Read the model definition and answer for the solid it produces. Units are mm, in the model's axes. A direction names the side the tool comes from. Coordinates: 2 decimals unless noted, no trailing zeros. Loops run counter-clockwise (first coordinate to the right, second up) from the corner with the lowest first, then second, coordinate; pieces in that order, holes last.
from build123d import *

# Parameters (mm, degrees)
SHELL1_T           = -0.8128
FILLET1_R          = 0.508
SKETCH3_W          = 0.762
SKETCH3_H          = 0.762
CUT_EXTRUDE1_DEPTH = 1.016


with BuildPart() as part:
    # Sketch1 → Revolve1 (revolve)
    with BuildSketch(Plane.XY, mode=Mode.PRIVATE) as revolve1_sk:
        with BuildLine():
            Line((0, 0), (0, 14.605))
            ThreePointArc((0, 14.605), (5.588, 14.065513703), (11.176, 14.605))
            Line((11.176, 14.605), (11.176, 0))
            Line((11.176, 0), (0, 0))
        make_face()
    revolve(revolve1_sk.sketch.rotate(Axis((-10.447687892, 0, 0), (1, 0, 0)), 90), axis=Axis((-10.447687892, 0, 0), (1, 0, 0)))

    # Shell1
    shell1_openings = [part.faces().sort_by_distance(p)[0] for p in [
        (0, 0, 0),
        (11.176, 0, 0),
    ]]
    offset(amount=SHELL1_T, openings=shell1_openings, kind=Kind.INTERSECTION)

    # Sketch2 → Revolve2 (revolve)
    with BuildSketch(Plane.XY, mode=Mode.PRIVATE) as revolve2_sk:
        with BuildLine():
            Line((8.636, 13.407835256), (8.636, 11.878888362))
            Line((8.636, 11.878888362), (10.922, 11.878888362))
            Line((10.922, 11.878888362), (10.922, 8.830888362))
            Line((10.922, 8.830888362), (14.732, 8.830888362))
            Line((14.732, 8.830888362), (14.732, 8.38570101))
            Line((14.732, 8.38570101), (10.805439867, 8.38570101))
            Line((10.805439867, 8.38570101), (10.805439867, 7.279783375))
            ThreePointArc((10.805439867, 7.279783375), (10.656650112, 6.92057313), (10.297439867, 6.771783375))
            Line((10.297439867, 6.771783375), (7.757439867, 6.771783375))
            Line((7.757439867, 6.771783375), (7.757439867, 7.279783375))
            Line((7.757439867, 7.279783375), (10.077783765, 7.279783375))
            ThreePointArc((10.077783765, 7.279783375), (10.233104084, 7.344119158), (10.297439867, 7.499439477))
            Line((10.297439867, 7.499439477), (10.297439867, 8.38570101))
            Line((10.297439867, 8.38570101), (6.741439867, 8.38570101))
            Line((6.741439867, 8.38570101), (6.741439867, 8.830888362))
            Line((6.741439867, 8.830888362), (10.297439867, 8.830888362))
            Line((10.297439867, 8.830888362), (10.297439867, 11.412306581))
            Line((10.297439867, 11.412306581), (8.128, 11.412306581))
            Line((8.128, 11.412306581), (8.128, 13.360351664))
            ThreePointArc((8.128, 13.360351664), (8.38210087, 13.383014307), (8.636, 13.407835256))
        make_face()
    revolve(revolve2_sk.sketch.rotate(Axis((-18.402780465, 0, 0), (1, 0, 0)), 90), axis=Axis((-18.402780465, 0, 0), (1, 0, 0)))

    # Fillet1
    fillet1_edges = [part.edges().sort_by_distance(p)[0] for p in [
        (10.922, 0, -11.878888362),
    ]]
    fillet(fillet1_edges, radius=FILLET1_R)

    # Sketch3 → Cut-Extrude1 (cut)
    with BuildSketch(Plane(origin=(10.805439867, 0, 0), x_dir=(0, 0, -1), z_dir=(1, 0, 0))):
        Polygon((4.038854556, 7.665935745), (3.657854556, 7.006024387), (4.317765913, 6.625024387), (4.698765913, 7.284935745), align=None)
        with Locations((0.045782775, 8.277322377)):
            Rectangle(SKETCH3_W, SKETCH3_H)
        Polygon((7.33071852, 4.619467821), (6.670807162, 4.238467821), (7.051807162, 3.578556464), (7.71171852, 3.959556464), align=None)
        with Locations((8.277322377, -0.045782775)):
            Rectangle(SKETCH3_W, SKETCH3_H)
        Polygon((7.665935745, -4.038854556), (7.006024387, -3.657854556), (6.625024387, -4.317765913), (7.284935745, -4.698765913), align=None)
        Polygon((4.619467821, -7.33071852), (4.238467821, -6.670807162), (3.578556464, -7.051807162), (3.959556464, -7.71171852), align=None)
        with Locations((-0.045782775, -8.277322377)):
            Rectangle(SKETCH3_W, SKETCH3_H)
        Polygon((-4.038854556, -7.665935745), (-3.657854556, -7.006024387), (-4.317765913, -6.625024387), (-4.698765913, -7.284935745), align=None)
        Polygon((-7.33071852, -4.619467821), (-6.670807162, -4.238467821), (-7.051807162, -3.578556464), (-7.71171852, -3.959556464), align=None)
        with Locations((-8.277322377, 0.045782775)):
            Rectangle(SKETCH3_W, SKETCH3_H)
        Polygon((-7.665935745, 4.038854556), (-7.006024387, 3.657854556), (-6.625024387, 4.317765913), (-7.284935745, 4.698765913), align=None)
        Polygon((-4.619467821, 7.33071852), (-4.238467821, 6.670807162), (-3.578556464, 7.051807162), (-3.959556464, 7.71171852), align=None)
    extrude(amount=-CUT_EXTRUDE1_DEPTH, mode=Mode.SUBTRACT)


solid = part.part
Q1. Determine the mould class of faces 1 (the face through (9.01, -6.714, -0.882)), 2 (the face through (14.732, 3, 8)) for opening direction Z: +Z half, -Z half, draft (parallel to the pull), parting line (faces both ways), or undercut.
Findings below:
face 1: undercut
face 2: draft
Q2. Flat-ended cylindrical pins translate along their axes: pin 1 Ø4 at (x, y) = (2, -6.5) entering from +Z; pin 2 Ø4 at (x, z) = (10.5, -3) entering from -Y; pin 3 Ø1.5 at (x, z) = (11, -11) entering from +Y. Find the tip coordinate at first contact, or state that the pin passes through.
Findings below:
pin 1: stops at z = 13.62
pin 2: stops at y = -14.56
pin 3: stops at y = 10.38
Q3. A cutting plane is placed at B-B (x = 13.5). Give the vertices of the cut face in (y, z).
Findings below:
outline: circle Ø17.66 at (0, 0); hole circle Ø16.77 at (0, 0)
Q4. Which of the six approach directions +Z, -Z, +X, -X, +Y, -Y give full straight-line access (tool end or side, diameter ignored) to faces 3 (the face through (9.537, 7.228, -9.427)), 4 (the face through (0, 11, 9)), 5 (the face through (8.54, 8.62, -1.91))?
Findings below:
face 3: +X
face 4: +Z, -Z, -X, +Y, -Y
face 5: -X
Q5. Straight lines are drawn through the part: probe 1 along Y at (x, z) = (13.6, 0); probe 2 along Y at (x, z) = (7.9, 0); probe 3 along Y at (x, z) = (11, -5.5). For each, find the intervals that lie inside material, in ascending order.
Findings below:
probe 1: y = -8.83 to -8.39, 8.39 to 8.83
probe 2: y = -14.16 to -13.34, -8.83 to -8.39, -7.28 to -6.77, 6.77 to 7.28, 8.39 to 8.83, 13.34 to 14.16
probe 3: y = -13.49 to -12.6, -6.91 to -6.33, 6.33 to 6.91, 12.6 to 13.49
Q6. A cutting plane is placed at A-A (x = 9). Give the vertices of the cut face in (y, z), then the cut area to 3 significant figures.
Findings below:
outline: circle Ø28.53 at (0, 0); circle Ø23.76 at (0, 0); circle Ø17.66 at (0, 0); circle Ø14.56 at (0, 0); hole circle Ø26.89 at (0, 0); hole circle Ø22.82 at (0, 0); hole circle Ø16.77 at (0, 0); hole circle Ø13.54 at (0, 0)
area: 152 mm2
